```python
from build123d import *

# Parameters (mm, degrees)
SKETCH1_R           = 1
SKETCH1_R_2         = 0.6
SKETCH1_R_3         = 2
BOSS_EXTRUDE1_DEPTH = 3
SKETCH3_R           = 0.8
CUT_EXTRUDE1_DEPTH  = 3
CIRPATTERN1_COUNT   = 6


with BuildPart() as part:
    # Sketch1 → Boss-Extrude1 (new body)
    with BuildSketch(Plane.XY):
        with BuildLine():
            Line((-23.1, 2), (-23.1, -6))
            Line((-23.1, -6), (-20.6, -6))
            Line((-20.6, -6), (-20.6, -5))
            ThreePointArc((-20.6, -5), (-20.307106781, -4.292893219), (-19.6, -4))
            Line((-19.6, -4), (-18.6, -4))
            ThreePointArc((-18.6, -4), (-17.892893219, -4.292893219), (-17.6, -5))
            Line((-17.6, -5), (-17.6, -6))
            Line((-17.6, -6), (3.4, -6))
            Line((3.4, -6), (3.4, -5))
            ThreePointArc((3.4, -5), (3.692893219, -4.292893219), (4.4, -4))
            Line((4.4, -4), (5.4, -4))
            ThreePointArc((5.4, -4), (6.107106781, -4.292893219), (6.4, -5))
            Line((6.4, -5), (6.4, -6))
            Line((6.4, -6), (15.9, -6))
            Line((15.9, -6), (15.9, 2))
            ThreePointArc((15.9, 2), (14.728427125, 4.828427125), (11.9, 6))
            Line((11.9, 6), (-19.1, 6))
            ThreePointArc((-19.1, 6), (-21.928427125, 4.828427125), (-23.1, 2))
        make_face()
        with Locations((-14, -3)):
            Circle(SKETCH1_R, mode=Mode.SUBTRACT)
        with Locations((12.9, -3)):
            Circle(SKETCH1_R, mode=Mode.SUBTRACT)
        with Locations((-19.1, 0)):
            Circle(SKETCH1_R_2, mode=Mode.SUBTRACT)
        with Locations((-14, 3)):
            Circle(SKETCH1_R, mode=Mode.SUBTRACT)
        with Locations((-4, 0)):
            Circle(SKETCH1_R_3, mode=Mode.SUBTRACT)
        with Locations((4.9, 0)):
            Circle(SKETCH1_R_2, mode=Mode.SUBTRACT)
        with Locations((12.9, 3)):
            Circle(SKETCH1_R, mode=Mode.SUBTRACT)
    extrude(amount=BOSS_EXTRUDE1_DEPTH)

    # Sketch3 → Cut-Extrude1 (cut)
    with BuildSketch(Plane.XY.offset(3)):
        with Locations((-4, 4.25)):
            Circle(SKETCH3_R)
    cut_extrude1 = extrude(amount=-CUT_EXTRUDE1_DEPTH, mode=Mode.SUBTRACT)

    # CirPattern1: Cut-Extrude1 ×6 about axis
    cirpattern1_axis = Axis((-4, 0, 0), (0, 0, 1))
    for i in range(1, CIRPATTERN1_COUNT):
        add(cut_extrude1.rotate(cirpattern1_axis, i * 360 / CIRPATTERN1_COUNT), mode=Mode.SUBTRACT)


solid = part.part
```
The model under review builds one solid part; all positions refer to its coordinate system, in mm. A direction names the side the tool comes from. Round coordinates to 2 decimals unless told otherwise and drop trailing zeros. Loops run counter-clockwise (first coordinate to the right, second up) from the corner with the lowest first, then second, coordinate; pieces in that order, holes last.
1) Consider section D-D on x = -14. State the section outline as (y, z) points, then the cut area to 3 significant figures.
Values follow:
outline: (-6, 0) - (-4, 0) - (-4, 3) - (-6, 3) - close; (-2, 0) - (2, 0) - (2, 3) - (-2, 3) - close; (4, 0) - (6, 0) - (6, 3) - (4, 3) - close
area: 24.0 mm2
2) Consider section C-C on x = 4.9. State the section outline as (y, z) points, then the cut area to 3 significant figures.
Values follow:
outline: (-4, 0) - (-0.6, 0) - (-0.6, 3) - (-4, 3) - close; (0.6, 0) - (6, 0) - (6, 3) - (0.6, 3) - close
area: 26.4 mm2
3) Wall thickness on line 1 along Y through (x, z) = (-4, 0.6); line 2 along Y through (x, z) = (-14, 2.4); line 3 along X through (y, z) = (-5.5, 2): over which ranges is each line inside the solid? List them lowest first.
Values follow:
line 1: y = -6 to -5.05, -3.45 to -2, 2 to 3.45, 5.05 to 6
line 2: y = -6 to -4, -2 to 2, 4 to 6
line 3: x = -23.1 to -20.6, -17.6 to 3.4, 6.4 to 15.9
4) Tool access review of faces 5 (the face through (3.4, -5.5, 1.5)), 6 (the face through (-21.897, 4.859, 1.479)): name each direction out of +Z, -Z, +X, -X, +Y, -Y from which nothing blocks a thin tool from reaching the whole face with its end or side.
Values follow:
face 5: +Z, -Z, -Y
face 6: +Z, -Z, -X, +Y
5) The part is to be moulded in two halves that separate along X. For faces 1 (the face through (-22, -6, 1)), 2 (the face through (6.099, -4.285, 1.479)), 3 (the face through (-23.1, -2, 1)), 4 (the face through (-8.05, 2.835, 1.521)), say which applies: pulls with the +X half, pulls with the -X half, needs draft (parallel to the pull), parting line crosses it, or undercut.
Values follow:
face 1: needs draft
face 2: undercut
face 3: pulls with the -X half
face 4: undercut
6) Clearance check with flat-ended pins moving along their axes: P1, Ø1, axis at x = -7.68, y = -2.12, coming from the -Z side; P2, Ø1.6, axis at x = -19.1, y = 0, coming from the +Z side; P3, Ø0.8, axis at x = 5, z = 1.5, coming from the -Y side. State where each tip first meets the part, or that it passes through.
Values follow:
P1: passes through
P2: stops at z = 3
P3: stops at y = -4
7) Consider section A-A on x = -4. State the section outline as (y, z) points, then the cut area to 3 significant figures.
Values follow:
outline: (-6, 0) - (-5.05, 0) - (-5.05, 3) - (-6, 3) - close; (-3.45, 0) - (-2, 0) - (-2, 3) - (-3.45, 3) - close; (2, 0) - (3.45, 0) - (3.45, 3) - (2, 3) - close; (5.05, 0) - (6, 0) - (6, 3) - (5.05, 3) - close
area: 14.4 mm2
8) Consider section B-B on y = 0. State the section outline as (x, z) points.
Values follow:
outline: (-23.1, 0) - (-19.7, 0) - (-19.7, 3) - (-23.1, 3) - close; (-18.5, 0) - (-6, 0) - (-6, 3) - (-18.5, 3) - close; (-2, 0) - (4.3, 0) - (4.3, 3) - (-2, 3) - close; (5.5, 0) - (15.9, 0) - (15.9, 3) - (5.5, 3) - close
